Work out the finished part from the listing and answer in its coordinate system (mm). A direction names the side the tool comes from. Give positions to 0.01 mm unless a question says otherwise; leave off trailing zeros. Order: outer loops, then holes, each group sorted by start corner. A loop starts at its lowest first (then second) coordinate and runs counter-clockwise, first axis right, second up. Notation, with made-up numbers: (62, -13) -> (115, -13) arc R16 ccw to (115, -2) -> close; hole circle Ø2 at (6, 53.25). An arc over 180 degrees is marked (long way). Use a Markdown table: item, result. Add a question column.
```python
from build123d import *

# Parameters (mm, degrees)
F1_DEPTH = 25.4


with BuildPart() as f1:
    # F0 (on Front) → F1 (new body)
    with BuildSketch(Plane.XZ):
        Polygon((-49.2131151259, 21.2018769234), (-56.0224764049, 21.2018769234), (-48.9432296743, 13.1197362788), (-45.1893992722, 8.8341129038), (-37.4514907598, 0), (42.0942343771, 0), (58.4986023605, 21.2018769234), (6.8093636073, 21.2018769234), (-3.4046829678, 21.2018769234), align=None)
        Polygon((-45.1893992722, 8.8341129038), (-48.9432296743, 13.1197362788), (-48.9432296743, 7.2736367583), (-56.9510273635, 7.2736367583), (-56.9510273635, -4.1784718633), (-45.1893992722, -4.1784718633), align=None)
        Polygon((-49.2131151259, 43.4870608151), (-49.2131151259, 21.2018769234), (-3.4046829678, 21.2018769234), (-4.7975066118, 32.3444688693), (-6.1903302558, 43.4870608151), (-31.8801924586, 43.4870608151), (-35.2848768234, 43.4870608151), align=None)
        Polygon((-4.7975066118, 32.3444688693), (-3.4046829678, 21.2018769234), (6.8093636073, 21.2018769234), align=None)
        with BuildLine():
            Line((-35.2848768234, 47.5522301825), (-35.2848768234, 43.4870608151))
            Line((-35.2848768234, 43.4870608151), (-31.8801924586, 43.4870608151))
            Line((-31.8801924586, 43.4870608151), (-31.8801924586, 49.0583635867))
            ThreePointArc((-31.8801924586, 49.0583635867), (-33.4234047275, 47.9455763399), (-35.2848768234, 47.5522301825))
        make_face()
        with BuildLine():
            ThreePointArc((-30.6835867198, 52.1535202861), (-38.5384802579, 55.4071237206), (-35.2848768234, 47.5522301825))
            Line((-35.2848768234, 47.5522301825), (-35.2848768234, 52.1535202861))
            Line((-35.2848768234, 52.1535202861), (-31.8801924586, 52.1535202861))
            Line((-31.8801924586, 52.1535202861), (-31.8801924586, 49.0583635867))
            ThreePointArc((-31.8801924586, 49.0583635867), (-30.9931515822, 50.4943141289), (-30.6835867198, 52.1535202861))
        make_face()
        with BuildLine():
            Line((-35.2848768234, 52.1535202861), (-35.2848768234, 47.5522301825))
            ThreePointArc((-35.2848768234, 47.5522301825), (-33.4234047275, 47.9455763399), (-31.8801924586, 49.0583635867))
            Line((-31.8801924586, 49.0583635867), (-31.8801924586, 52.1535202861))
            Line((-31.8801924586, 52.1535202861), (-35.2848768234, 52.1535202861))
        make_face()
    extrude(amount=F1_DEPTH)


solid = f1.part
```
1) Determine the mould class of faces 1 (the flat face through (-42, -13, 43.487)), 2 (the flat face through (33, -13, 21.202)), 3 (the flat face through (-51, -13, -4.178)), 4 (the flat face through (-45.189, -13, 2)) for opening direction Z: released by +Z, released by -Z, zero draft, split by the parting line, or undercut.
2) Straight lines are drawn through the part: line 1 (Z direction, x = -17, y = -21.5); line 2 (X direction, y = -5.5, z = 1); line 3 (X direction, y = -15.75, z = 45.5). For each, find the intervals that lie inside material, in ascending order.
3) Flat-ended cylindrical pins translate along their axes: pin 1 (10 mm diameter, centred on x = -35, z = 39.5, fed in from +Y); pin 2 (2.5 mm diameter, centred on x = -53, y = -13.5, fed in from +Z); pin 3 (6.5 mm diameter, centred on y = -17.5, z = 5.5, fed in from +X); pin 4 (1.7 mm diameter, centred on y = -18.5, z = 46, fed in from +X). Find the tip coordinate at first contact, or state that the pin passes through.
4) The part is cut by section C-C, the plane z = 40. Determine the outline of the cut face in (x, y), then the cut area to 3 significant figures.
5) Which of the six approach directions +Z, -Z, +X, -X, +Y, -Y give full straight-line access (tool end or side, diameter ignored) to faces 5 (the flat face through (-53, -13, 21.202)), 6 (the flat face through (-53, -13, 7.274)), 7 (the flat face through (-41.375, -12.522, 4.479))?
6) The part is cut by section B-B, the plane x = -14. Determine the outline of the cut face in (y, z), then the cut area to 3 significant figures.
7) The part is cut by section A-A, the plane y = -17.75. Determine the outline of the cut face in (x, z).
A:
| question | item | result |
|---|---|---|
| 1 | face 1 | undercut |
| 1 | face 2 | released by +Z |
| 1 | face 3 | released by -Z |
| 1 | face 4 | zero draft |
| 2 | line 1 | 0 to 43.49 |
| 2 | line 2 | -56.95 to -45.19, -38.33 to 42.87 |
| 2 | line 3 | -35.28 to -31.88 |
| 3 | pin 1 | y = 0 |
| 3 | pin 2 | z = 21.2 |
| 3 | pin 3 | x = 48.86 |
| 3 | pin 4 | x = -31.88 |
| 4 | outline | (-49.21, -25.4) -> (-5.75, -25.4) -> (-5.75, 0) -> (-49.21, 0) -> close |
| 4 | area | 1,100 mm^2 |
| 5 | face 5 | +Z, -X, +Y, -Y |
| 5 | face 6 | -X, +Y, -Y |
| 5 | face 7 | -Z, +Y, -Y |
| 6 | outline | (-25.4, 0) -> (0, 0) -> (0, 43.49) -> (-25.4, 43.49) -> close |
| 6 | area | 1,100 mm^2 |
| 7 | outline | (-56.95, -4.18) -> (-45.19, -4.18) -> (-45.19, 8.83) -> (-37.45, 0) -> (42.09, 0) -> (58.5, 21.2) -> (6.81, 21.2) -> (-4.8, 32.34) -> (-6.19, 43.49) -> (-31.88, 43.49) -> (-31.88, 49.06) arc R4.6 ccw (long way) to (-35.28, 47.55) -> (-35.28, 43.49) -> (-49.21, 43.49) -> (-49.21, 21.2) -> (-56.02, 21.2) -> (-48.94, 13.12) -> (-48.94, 7.27) -> (-56.95, 7.27) -> close |
